from build123d import *

# Parameters (mm, degrees)
SKETCH068_W            = 9
SKETCH068_H            = 275
PAD022_DEPTH           = 6.5
SKETCH067_R            = 1.5
POCKET041_DEPTH        = 6.5
LINEARPATTERN009_COUNT = 14
LINEARPATTERN009_PITCH = 20


with BuildPart() as part:
    # Sketch068 → Pad022 (new body)
    with BuildSketch(Plane.XY):
        with Locations((-4.5, 137.5)):
            Rectangle(SKETCH068_W, SKETCH068_H)
    extrude(amount=PAD022_DEPTH)

    # Sketch067 (on Face6 of Pad022) → Pocket041 (cut)
    with BuildSketch(Plane.XY.offset(6.5)):
        with Locations((-4.5, 7.5)):
            Circle(SKETCH067_R)
    pocket041 = extrude(amount=-POCKET041_DEPTH, mode=Mode.SUBTRACT)

    # LinearPattern009: Pocket041 ×14
    with Locations(*[(0, i * LINEARPATTERN009_PITCH, 0) for i in range(1, LINEARPATTERN009_COUNT)]):
        add(pocket041, mode=Mode.SUBTRACT)


solid = part.part
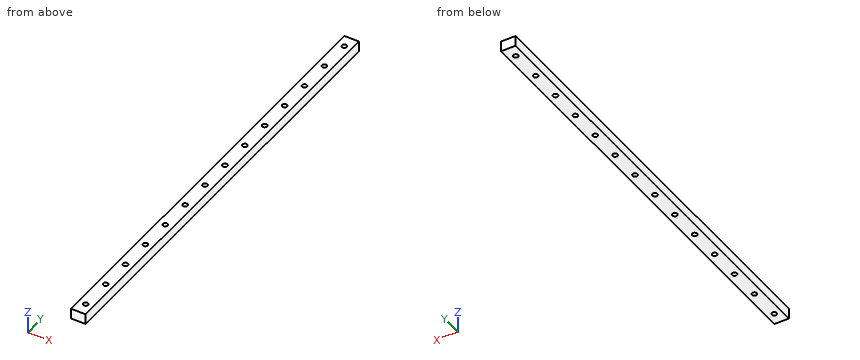
Source: CAD feature listing. Evaluate the final solid. Frame: model axes, mm. Coordinates: 2 decimals unless noted, no trailing zeros. Use a Markdown table: item, result.
1) Section A-A, the plane z = 4.5. Give the number of separate pieces and of enclosed holes in the cut face, then the cut area to 3 significant figures.
Conclusion:
| item | result |
|---|---|
| separate pieces | 1 |
| enclosed holes | 14 |
| area | 2,380 mm^2 |
2) First-contact query: pin 1 Ø2.5 at (x, y) = (-4.5, 167.5) entering from +Z. Flat tip, straight axial feed; report the tip coordinate or a pass-through.
Conclusion:
| item | result |
|---|---|
| pin 1 | passes through |
3) Ray query, L1, parallel to X at y = 247.5, z = 4.25; L2, parallel to X at y = 188.5, z = 5.25. Return the intervals inside material, ascending.
Conclusion:
| item | result |
|---|---|
| L1 | x = -9 to -6, -3 to 0 |
| L2 | x = -9 to -5.62, -3.38 to 0 |
